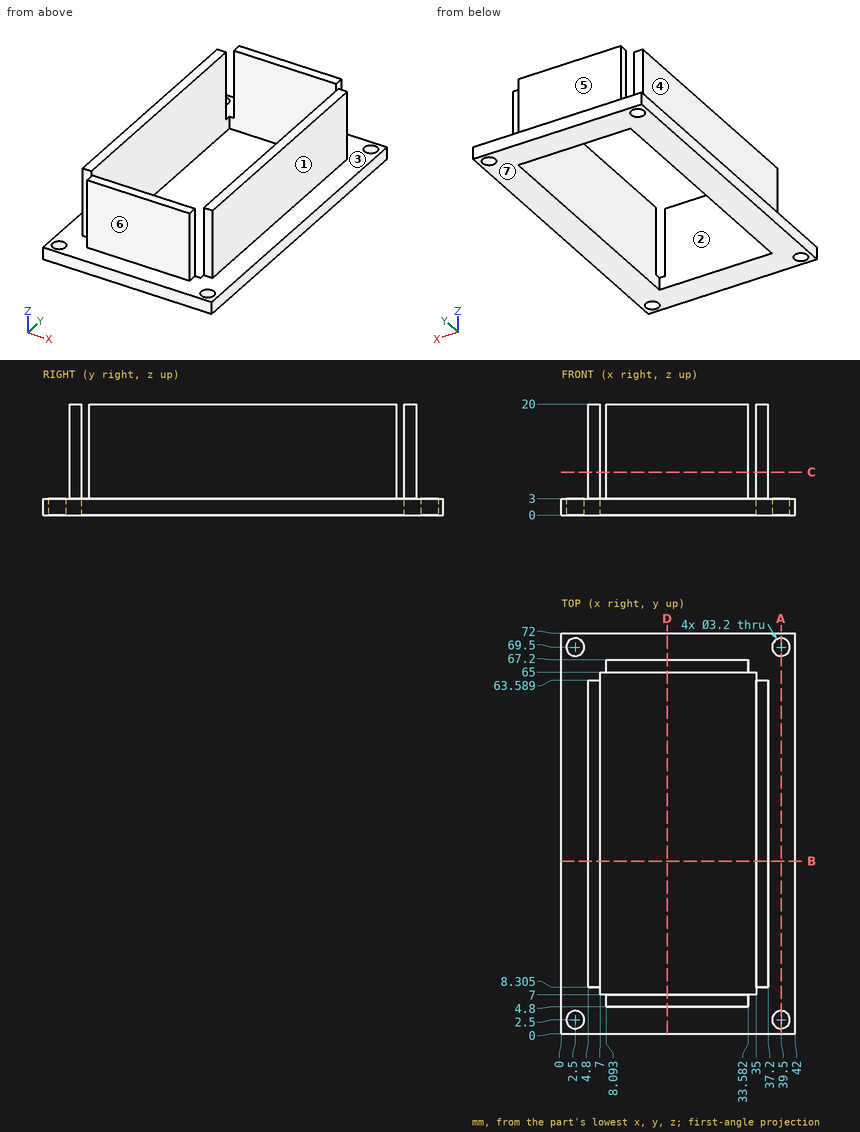
Design review of the part shown in the three views and the two pictorial views. Dimensions are in mm from the part's minimum x, y and z. A direction names the side the tool comes from. Give positions to 0.01 mm unless a question says otherwise; leave off trailing zeros. Loops run counter-clockwise (first coordinate to the right, second up) from the corner with the lowest first, then second, coordinate; pieces in that order, holes last. Notation, with made-up numbers: M -28,20 L -20,20 A14 cw -20,29 Z; hole C 39,74 d1. An arc over 180 degrees is marked long. Answer as a JSON object with one key per item and string values.
Item 1: We need section C-C (z = 7.75). State the section outline as (x, y) points (1 decimal).
Output values:
{"outline": "M 4.8,8.3 L 7,8.3 L 7,63.6 L 4.8,63.6 Z; M 8.1,4.8 L 33.6,4.8 L 33.6,7 L 8.1,7 Z; M 8.1,65 L 33.6,65 L 33.6,67.2 L 8.1,67.2 Z; M 35,8.3 L 37.2,8.3 L 37.2,63.6 L 35,63.6 Z"}
Item 2: For P1, Ø1.8, axis at x = 35.5, z = 10, coming from the +Y side; P2, Ø3, axis at x = 35, z = 16, coming from the -Y side; P3, Ø6, axis at x = 31, y = 31.5, coming from the +Z side; P4, Ø2.5, axis at y = 5.5, z = 8, coming from the +X side, all flat-tipped, find the tip position at first contact; note any pin that passes through.
Output values:
{"P1": "stops at y = 63.59", "P2": "stops at y = 4.8", "P3": "passes through", "P4": "stops at x = 33.58"}
Item 3: We need section A-A (x = 39.5). State the section outline as (y, z) points, and give its area (3 significant figures).
Output values:
{"outline": "M 0,0 L 0.9,0 L 0.9,3 L 0,3 Z; M 4.1,0 L 67.9,0 L 67.9,3 L 4.1,3 Z; M 71.1,0 L 72,0 L 72,3 L 71.1,3 Z", "area": "197 mm2"}
Item 4: Wall thickness on line 1 along Y through (x, z) = (39.5, 1.2); line 2 along X through (y, z) = (69.5, 1.4); line 3 along X through (y, z) = (17.5, 12.5): over which ranges is each line inside the solid? List them lowest first.
Output values:
{"line 1": "y = 0 to 0.9, 4.1 to 67.9, 71.1 to 72", "line 2": "x = 0 to 0.9, 4.1 to 37.9, 41.1 to 42", "line 3": "x = 4.8 to 7, 35 to 37.2"}
Item 5: We need section D-D (x = 19). State the section outline as (y, z) points.
Output values:
{"outline": "M 0,0 L 7,0 L 7,20 L 4.8,20 L 4.8,3 L 0,3 Z; M 65,0 L 72,0 L 72,3 L 67.2,3 L 67.2,20 L 65,20 Z"}
Item 6: We need section B-B (y = 31). State the section outline as (x, z) points.
Output values:
{"outline": "M 0,0 L 7,0 L 7,20 L 4.8,20 L 4.8,3 L 0,3 Z; M 35,0 L 42,0 L 42,3 L 37.2,3 L 37.2,20 L 35,20 Z"}
Item 7: Machinability: for the marked faces 5, 6 and 7, which of the approach directions +Z, -Z, +X, -X, +Y, -Y give a long, thin tool a straight path to every point of the face, cutting with its end or side? Answer none if there is none.
Output values:
{"face 5": "+Z, +X, -X, +Y", "face 6": "+Z, +X, -X, -Y", "face 7": "-Z, +X, -X, +Y, -Y"}
Item 8: Mouldability with a two-part tool opening along X and no side actions: class the marked faces 1, 2, 3 and 4 as pulls with the +X half, pulls with the -X half, needs draft (parallel to the pull), parting line crosses it, or undercut.
Output values:
{"face 1": "pulls with the +X half", "face 2": "undercut", "face 3": "needs draft", "face 4": "pulls with the -X half"}
